The model under review builds one solid part; all positions refer to its coordinate system, in mm. A direction names the side the tool comes from. Round coordinates to 2 decimals unless told otherwise and drop trailing zeros. Loops run counter-clockwise (first coordinate to the right, second up) from the corner with the lowest first, then second, coordinate; pieces in that order, holes last. Notation, with made-up numbers: (87.25, 71.25) -> (107.25, 71.25) arc R4 cw to (107.25, 76.25) -> close; hole circle Ø4 at (42.25, 4). An arc over 180 degrees is marked (long way). Write each question's results on one line, items separated by ' | '. Start each with the question number.
Item 1: We need section A-A (y = 19). Give the boundary of the cut face in (x, z).
Item 2: We need section B-B (z = -3). Give the boundary of the cut face in (x, y).
Item 3: For L1, parallel to Y at x = -4, z = -8.75; L2, parallel to X at y = 41.5, z = -3.75; L3, parallel to Z at x = 1.25, y = 33, list the stretches that pass through material, from the lowest coordinate up. Write a range as from..to.
Item 4: Tool access review of faces 5 (the flat face through (12, 57, -4)), 6 (the cylindrical face through (9.55, -1.34, -13.61)), 7 (the flat face through (0, 0, -6)), 8 (the cylindrical face through (-9.47, 58.32, -13.76)), 9 (the flat face through (0, -1, -12.2)): name each direction out of +Z, -Z, +X, -X, +Y, -Y from which nothing blocks a thin tool from reaching the whole face with its end or side.
Item 5: Clearance check with flat-ended pins moving along their axes: pin 1 Ø2 at (y, z) = (-1, -11) entering from +X; pin 2 Ø0.5 at (x, z) = (13, -4) entering from +Y; pin 3 Ø1.5 at (x, y) = (4.5, 26.5) entering from +Z. State where each tip first meets the part, or that it passes through.
Item 6: Mouldability with a two-part tool opening along Z and no side actions: class faces 1 (the flat face through (0, 57, -11)), 2 (the flat face through (3.95, -1, -11)), 3 (the flat face through (0, 28, -17)), 4 (the flat face through (0, -1, -9)) as pulls with the +Z half, pulls with the -Z half, needs draft (parallel to the pull), parting line crosses it, or undercut.
from build123d import *

# Parameters (mm, degrees)
BOSS_EXTRUDE1_DEPTH = 57
SKETCH4_W           = 6.5
SKETCH4_H           = 8.5
CUT_EXTRUDE1_DEPTH  = 62.236345417
BOSS_EXTRUDE2_DEPTH = 1.8
SKETCH5_W           = 7.9
SKETCH5_H           = 3.2
CUT_EXTRUDE2_DEPTH  = 63.91526047
BOSS_EXTRUDE3_DEPTH = 1.8
FILLET1_R           = 1.6


with BuildPart() as part:
    # Sketch1 → Boss-Extrude1 (new body)
    with BuildSketch(Plane(origin=(0, 0, 0), x_dir=(1, 0, 0), z_dir=(0, 1, 0))):
        Polygon((11.5, 0), (11.5, 9), (10.5, 9), (10.5, 10.454545455), (6, 17), (-6, 17), (-10.5, 10.454545455), (-10.5, 9), (-11.5, 9), (-11.5, 0), (-13.3, 0), (-13.3, 9), (-7.331417468, 17.681574593), (-7.1125, 18), (7.1125, 18), (7.368594903, 17.627498323), (13.3, 9), (13.3, 0), align=None)
    extrude(amount=BOSS_EXTRUDE1_DEPTH)

    # Sketch4 → Cut-Extrude1 (cut, through all)
    with BuildSketch(Plane(origin=(0, 0, -18), x_dir=(-1, 0, 0), z_dir=(0, 0, -1))):
        with Locations((-2.45, 12.45)):
            Rectangle(SKETCH4_W, SKETCH4_H)
    extrude(amount=-CUT_EXTRUDE1_DEPTH, mode=Mode.SUBTRACT)

    # Sketch2 → Boss-Extrude2 (add)
    with BuildSketch(Plane.XZ):
        Polygon((-13.3, 0), (-13.3, -9), (-7.1125, -18), (7.1125, -18), (13.3, -9), (13.3, 0), align=None)
    extrude(amount=BOSS_EXTRUDE2_DEPTH)

    # Sketch5 → Cut-Extrude2 (cut, through all)
    with BuildSketch(Plane.XZ.offset(1.8)):
        with Locations((0, -10.6)):
            Rectangle(SKETCH5_W, SKETCH5_H)
    extrude(amount=-CUT_EXTRUDE2_DEPTH, mode=Mode.SUBTRACT)

    # Sketch3 → Boss-Extrude3 (add)
    with BuildSketch(Plane(origin=(0, 57, 0), x_dir=(1, 0, 0), z_dir=(0, 1, 0))):
        Polygon((-13.3, 9), (-7.1125, 18), (7.1125, 18), (13.3, 9), (13.3, 7), (-13.3, 7), align=None)
    extrude(amount=BOSS_EXTRUDE3_DEPTH)

    # Fillet1
    fillet1_edges = [part.edges().sort_by_distance(p)[0] for p in [
        (-13.3, 58.8, -8),
        (13.3, 58.8, -8),
        (10.20625, 58.8, -13.5),
        (-10.20625, 58.8, -13.5),
        (-13.3, -1.8, -4.5),
        (-10.20625, -1.8, -13.5),
        (10.20625, -1.8, -13.5),
        (13.3, -1.8, -4.5),
    ]]
    fillet(fillet1_edges, radius=FILLET1_R)


solid = part.part
Here are the results:
1) outline: (-13.3, -9) -> (-7.11, -18) -> (7.11, -18) -> (13.3, -9) -> (13.3, 0) -> (11.5, 0) -> (11.5, -9) -> (10.5, -9) -> (10.5, -10.45) -> (6, -17) -> (-6, -17) -> (-10.5, -10.45) -> (-10.5, -9) -> (-11.5, -9) -> (-11.5, 0) -> (-13.3, 0) -> close
2) outline: (-13.3, -0.2) arc R1.6 ccw to (-11.7, -1.8) -> (11.7, -1.8) arc R1.6 ccw to (13.3, -0.2) -> (13.3, 57) -> (11.5, 57) -> (11.5, 0) -> (-11.5, 0) -> (-11.5, 57) -> (-13.3, 57) -> close
3) L1: y = -1.8..0, 57..58.8 | L2: x = -13.3..-11.5, 11.5..13.3 | L3: z = -18..-17
4) face 5: +Z, +X, -X, +Y | face 6: -Z, +X, -Y | face 7: +Z | face 8: -Z, -X, +Y | face 9: -Y
5) pin 1: stops at x = 12.49 | pin 2: stops at y = 57 | pin 3: stops at z = -17
6) face 1: needs draft | face 2: undercut | face 3: pulls with the +Z half | face 4: undercut
